from build123d import *

# Parameters (mm, degrees)
SKETCH1_R           = 3.1
BOSS_EXTRUDE1_DEPTH = 42.5
SKETCH2_R           = 10.1
SKETCH2_R_2         = 5.1
BOSS_EXTRUDE2_DEPTH = 52.5
CUT_EXTRUDE1_DEPTH  = 42.5


with BuildPart() as part:
    # Sketch1 → Boss-Extrude1 (new body)
    with BuildSketch(Plane(origin=(0, 0, 0), x_dir=(1, 0, 0), z_dir=(0, 1, 0))):
        Polygon((-50, 25.25), (-50, 5.5), (-45, 7.5), (-45, -7.5), (-50, -5.5), (-50, -25.25), (50, -25.25), (50, -5.5), (45, -7.5), (45, 7.5), (50, 5.5), (50, 25.25), align=None)
        with Locations(Location((0, 0, 0), (0, 0, 270))):
            Circle(SKETCH1_R, mode=Mode.SUBTRACT)
    extrude(amount=BOSS_EXTRUDE1_DEPTH)

    # Sketch2 → Boss-Extrude2 (add)
    with BuildSketch(Plane(origin=(0, 42.5, 0), x_dir=(1, 0, 0), z_dir=(0, 1, 0))):
        with Locations(Location((0, 0, 0), (0, 0, 270))):
            Circle(SKETCH2_R)
        with Locations(Location((0, 0, 0), (0, 0, 270))):
            Circle(SKETCH2_R_2, mode=Mode.SUBTRACT)
    extrude(amount=BOSS_EXTRUDE2_DEPTH)

    # Sketch3 → Cut-Extrude1 (cut)
    with BuildSketch(Plane(origin=(0, 42.5, 0), x_dir=(1, 0, 0), z_dir=(0, 1, 0))):
        Polygon((-37.5, -17.75), (-37.5, 17.75), (-7.5, 17.75), (-15, 3.769353064), (-15, -3.769353064), (-7.5, -17.75), align=None)
        Polygon((15, -3.769353064), (7.5, -17.75), (37.5, -17.75), (37.5, 17.75), (7.5, 17.75), (15, 3.769353064), align=None)
    extrude(amount=-CUT_EXTRUDE1_DEPTH, mode=Mode.SUBTRACT)


solid = part.part
Could you check a few things on this model? Use its own coordinates, in mm. A direction names the side the tool comes from. Give positions to 0.01 mm unless a question says otherwise; leave off trailing zeros. Write each loop counter-clockwise with the first axis right and the second up, starting at its lowest first coordinate (ties: lowest second). Pieces come first, ordered by that corner, then holes. Notation, with made-up numbers: (-18.5, 58.25) -> (-1.5, 58.25) arc R21 ccw to (-1.5, 96.25) -> close; hole circle Ø3 at (74, 24). An arc over 180 degrees is marked (long way). Answer as a JSON object with one key per item and string values.
Q1. Which directions (+Z, -Z, +X, -X, +Y, -Y) give clear straight access to the entire face, cutting with the end or side of a thin tool? Please do faces 4 (the flat face through (2, 95, -5)), 5 (the flat face through (15, 22, 0)).
Taken from the geometry:
{"face 4": "+Z, -Z, +X, -X, +Y", "face 5": "+Y, -Y"}
Q2. Please list where these lines run through material, in increasing order: L1, parallel to X at y = 23, z = 0; L2, parallel to X at y = 40, z = 10; L3, parallel to Z at x = 37, y = 19.5.
Taken from the geometry:
{"L1": "x = -45 to -37.5, -15 to -3.1, 3.1 to 15, 37.5 to 45", "L2": "x = -50 to -37.5, -11.66 to 11.66, 37.5 to 50", "L3": "z = -25.25 to -17.75, 17.75 to 25.25"}
Q3. Suppose I cut it at A-A on z = 0. Write out the boundary of the cut face in (x, y), then the cut area to 3 significant figures.
Taken from the geometry:
{"outline": "(-45, 0) -> (-37.5, 0) -> (-37.5, 42.5) -> (-45, 42.5) -> close; (-15, 0) -> (-3.1, 0) -> (-3.1, 42.5) -> (-5.1, 42.5) -> (-5.1, 95) -> (-10.1, 95) -> (-10.1, 42.5) -> (-15, 42.5) -> close; (3.1, 0) -> (15, 0) -> (15, 42.5) -> (10.1, 42.5) -> (10.1, 95) -> (5.1, 95) -> (5.1, 42.5) -> (3.1, 42.5) -> close; (37.5, 0) -> (45, 0) -> (45, 42.5) -> (37.5, 42.5) -> close", "area": "2,170 mm²"}
Q4. Suppose I cut it at B-B on x = 0. Write out the boundary of the cut face in (y, z).
Taken from the geometry:
{"outline": "(0, -25.25) -> (42.5, -25.25) -> (42.5, -10.1) -> (95, -10.1) -> (95, -5.1) -> (42.5, -5.1) -> (42.5, -3.1) -> (0, -3.1) -> close; (0, 3.1) -> (42.5, 3.1) -> (42.5, 5.1) -> (95, 5.1) -> (95, 10.1) -> (42.5, 10.1) -> (42.5, 25.25) -> (0, 25.25) -> close"}
Q5. We'd pull the mould along Z, two halves only. Please class faces 1 (the flat face through (-45, 21, 0)), 2 (the flat face through (50, 21, 16)), 3 (the flat face through (-1, 21, 25.25)): released by +Z, released by -Z, zero draft, split by the parting line, or undercut.
Taken from the geometry:
{"face 1": "undercut", "face 2": "zero draft", "face 3": "released by +Z"}
Q6. Will these pins go through, and if not, where does the flat tip stop? pin 1 Ø2.5 at (y, z) = (22, -1) entering from -X; pin 2 Ø12 at (x, z) = (-20.5, -3.5) entering from +Y; pin 3 Ø8.5 at (y, z) = (13.5, -0.5) entering from +X.
Taken from the geometry:
{"pin 1": "stops at x = -45", "pin 2": "stops at y = 42.5", "pin 3": "stops at x = 45"}
Q7. Suppose I cut it at D-D on z = -12.5. Write out the boundary of the cut face in (x, y).
Taken from the geometry:
{"outline": "(-50, 0) -> (-37.5, 0) -> (-37.5, 42.5) -> (-50, 42.5) -> close; (-10.32, 0) -> (10.32, 0) -> (10.32, 42.5) -> (-10.32, 42.5) -> close; (37.5, 0) -> (50, 0) -> (50, 42.5) -> (37.5, 42.5) -> close"}
Q8. Suppose I cut it at C-C on y = 33. Write out the boundary of the cut face in (x, z).
Taken from the geometry:
{"outline": "(-50, -25.25) -> (50, -25.25) -> (50, -5.5) -> (45, -7.5) -> (45, 7.5) -> (50, 5.5) -> (50, 25.25) -> (-50, 25.25) -> (-50, 5.5) -> (-45, 7.5) -> (-45, -7.5) -> (-50, -5.5) -> close; hole (-37.5, -17.75) -> (-7.5, -17.75) -> (-15, -3.77) -> (-15, 3.77) -> (-7.5, 17.75) -> (-37.5, 17.75) -> close; hole circle Ø6.2 at (0, 0); hole (7.5, -17.75) -> (37.5, -17.75) -> (37.5, 17.75) -> (7.5, 17.75) -> (15, 3.77) -> (15, -3.77) -> close"}
